Model file for the job. Use its own axes, mm. Face numbers are marked on the shaded views. Give positions to 0.01 mm unless a question says otherwise; leave off trailing zeros. Write each loop counter-clockwise with the first axis right and the second up, starting at its lowest first coordinate (ties: lowest second). Pieces come first, ordered by that corner, then holes.
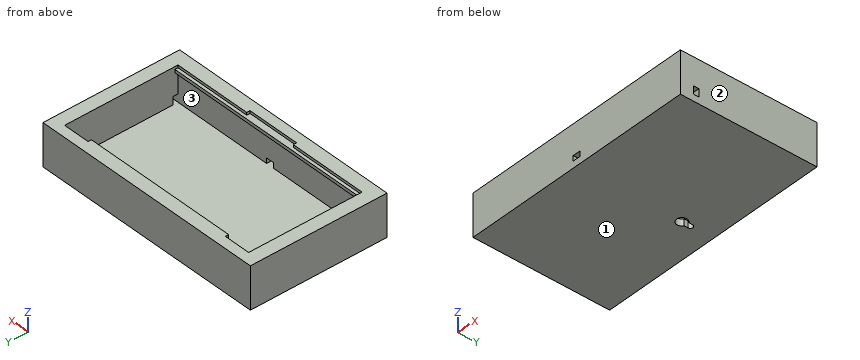
Autodesk Inventor part; units mm, degrees
ref_plane "YZ Plane" through (0, 0, 0) normal (1, 0, 0) x (0, 1, 0)
ref_plane "XZ Plane" through (0, 0, 0) normal (0, 1, 0) x (-1, 0, 0)
ref_plane "XY Plane" through (0, 0, 0) normal (0, 0, 1) x (1, 0, 0)
sketch "Sketch1" plane through (0, 0, 0) normal (0, 0, 1) x (1, 0, 0)
  line L0 (-100, -52.5) -> (100, -52.5)
  line L1 (100, -52.5) -> (100, 52.5)
  line L2 (100, 52.5) -> (-100, 52.5)
  line L3 (-100, 52.5) -> (-100, -52.5)
  line L4 (-100, -52.5) -> (100, 52.5) construction
  line L5 (100, -52.5) -> (-100, 52.5) construction
  line L6 (-112.7, 65.2) -> (112.7, 65.2)
  line L7 (112.7, 65.2) -> (112.7, -65.2)
  line L8 (112.7, -65.2) -> (-112.7, -65.2)
  line L9 (-112.7, -65.2) -> (-112.7, 65.2)
  point P0 (0, 0)
  dimension "d0" = 200
  dimension "d1" = 105
  dimension "d2" = 12.7
extrude "Extrusion1" add sketch "Sketch1" against normal blind 40
sketch "Sketch2" plane through (-100, 52.5, 0) normal (0, -1, 0) x (1, 0, 0)
  line L0 (200, -40) -> (0, -40)
  line L1 (0, 0) -> (0, -40)
  line L2 (200, -40) -> (0, -40)
  line L3 (0, -40) -> (0, -33.65)
  line L4 (0, -33.65) -> (200, -33.65)
  line L5 (200, -33.65) -> (200, -40)
  point P0 (100, 0)
  dimension "d5" = 6.35
extrude "Extrusion2" add sketch "Sketch2" along normal up to next
sketch "Sketch4" plane through (0, 0, -40) normal (0, 0, -1) x (-1, 0, 0)
  line L0 (112.7, 65.2) -> (-112.7, 65.2)
  line L1 (0, 65.2) -> (0, -65.2)
  line L2 (-112.7, -65.2) -> (112.7, -65.2)
  arc A0 (-2.5, 39.5301) -> (2.5, 39.5301) centre (0, 35.2) ccw
  line L3 (0, 35.2) -> (0, 43.2) construction
  line L4 (2.5, 39.5301) -> (2.5, 43.2)
  line L5 (-2.5, 43.2) -> (-2.5, 39.5301)
  arc A1 (2.5, 43.2) -> (-2.5, 43.2) centre (0, 43.2) ccw
  point P0 (0, 0)
  point P1 (0, 39.2)
  dimension "d14" = 10
  dimension "d15" = 5
  dimension "d17" = 30
  dimension "d18" = 8
extrude "Extrusion4" cut sketch "Sketch4" against normal through all
sketch "Sketch5" plane through (100, -52.5, 0) normal (-1, 0, 0) x (0, 0, 1)
  line L0 (-33.65, 105) -> (-33.65, 0)
  line L1 (0, 0) -> (-40, 0)
  line L2 (-33.65, 0) -> (-26.15, 0)
  line L3 (-26.15, 0) -> (-26.15, 5)
  line L4 (-26.15, 5) -> (-33.65, 5)
  line L5 (-33.65, 5) -> (-33.65, 0)
  point P0 (0, 52.5)
  dimension "d21" = 7.5
  dimension "d22" = 5
extrude "Extrusion5" cut sketch "Sketch5" against normal through all
sketch "Sketch6" plane through (-100, -52.5, 0) normal (1, 0, 0) x (0, 0, -1)
  line L0 (0, 0) -> (33.65, 0)
  line L1 (0, 0) -> (0, 105)
  line L2 (0, 105) -> (33.65, 105)
  line L3 (2.5, 0) -> (5.5, 0)
  line L4 (5.5, 0) -> (5.5, 3)
  line L5 (5.5, 3) -> (2.5, 3)
  line L6 (2.5, 3) -> (2.5, 0)
  point P0 (0, 52.5)
  point P1 (40, 0)
  point P2 (40, 105)
  dimension "d26" = 2.5
  dimension "d27" = 3
  dimension "d28" = 3
extrude "Extrusion6" add sketch "Sketch6" along normal up to next
sketch "Sketch7" plane through (0, 0, 0) normal (0, 0, 1) x (1, 0, 0)
  line L0 (112.7, -65.2) -> (-112.7, -65.2)
  line L1 (0, -65.2) -> (0, -52.5)
  line L2 (-100, -52.5) -> (112.7, -52.5)
  line L3 (-25.4, -55.675) -> (25.4, -55.675)
  line L4 (25.4, -55.675) -> (25.4, -52.5)
  line L5 (25.4, -52.5) -> (-25.4, -52.5)
  line L6 (-25.4, -52.5) -> (-25.4, -55.675)
  line L7 (-25.4, -55.675) -> (25.4, -52.5) construction
  line L8 (25.4, -55.675) -> (-25.4, -52.5) construction
  arc A0 (25.4, -55.675) -> (28.575, -52.5) centre (25.4, -52.5) ccw construction
  arc A1 (-28.575, -52.5) -> (-25.4, -55.675) centre (-25.4, -52.5) ccw construction
  point P0 (0, 0)
  point P1 (0, -54.0875)
  point P2 (100, -52.5)
  dimension "d32" = 50.8
  dimension "d33" = 3.175
extrude "Extrusion7" cut sketch "Sketch7" against normal up to surface (2.5 mm away)
sketch "Sketch8" plane through (0, 0, 0) normal (0, 0, 1) x (1, 0, 0)
  line L0 (-100, -52.5) -> (-100, 52.5)
  line L1 (-100, 52.5) -> (-74.6, 52.5)
  line L2 (-74.6, 52.5) -> (-74.6, 55.675)
  line L3 (-74.6, 55.675) -> (-100, 55.675)
  line L4 (-100, 55.675) -> (-100, 52.5)
  point P0 (0, 0)
  dimension "d36" = 25.4
  dimension "d37" = 3.175
extrude "Extrusion8" cut sketch "Sketch8" against normal blind 22.86
mirror "Mirror1" about plane through (0, 0, 0) normal (1, 0, 0) of "Extrusion8"
sketch "Sketch9" plane through (-100, -52.5, -33.65) normal (0, 1, 0) x (1, 0, 0)
  line L0 (0, 0) -> (212.7, 0)
  line L1 (96.2535, -5.0038) -> (103.7465, -5.0038)
  line L2 (103.7465, -5.0038) -> (103.7465, 0)
  line L3 (103.7465, 0) -> (96.2535, 0)
  line L4 (96.2535, 0) -> (96.2535, -5.0038)
  line L5 (212.7, 6.35) -> (-12.7, 6.35)
  line L6 (100, 6.35) -> (100, -33.65)
  line L7 (125.4, -33.65) -> (74.6, -33.65)
  point P0 (100, 0)
  point P1 (200, 0)
  dimension "d40" = 7.493
  dimension "d41" = 5.0038
extrude "Extrusion9" cut sketch "Sketch9" against normal through all
properties part number "housing"
1. Pull direction X, two halves, no side cores. Call the marked faces 1, 2 and 3: +X half, -X half, draft (parallel to the pull), parting line (faces both ways), or undercut.
Calculated:
face 1: draft
face 2: +X half
face 3: undercut
2. Slice it at B-B, the plane z = -9. Write the cut outline in (x, y) (3 decimals).
Calculated:
outline: (-112.7, -65.2) - (112.7, -65.2) - (112.7, 65.2) - (-112.7, 65.2) - close; hole (-100, -52.5) - (100, -52.5) - (100, 55.675) - (74.6, 55.675) - (74.6, 52.5) - (-74.6, 52.5) - (-74.6, 55.675) - (-100, 55.675) - close
3. Slice it at C-C, the plane y = -9.5. Write the cut outline in (x, z).
Calculated:
outline: (-112.7, -40) - (112.7, -40) - (112.7, 0) - (100, 0) - (100, -33.65) - (-100, -33.65) - (-100, 0) - (-112.7, 0) - close
4. Probe probe 1 along Y at (x, z) = (0, -35.25); probe 2 along X at (y, z) = (6, -19.5); probe 3 along Y at (x, z) = (94, -27.5). List the from-to ranges inside material, lowest first.
Calculated:
probe 1: y = -65.2 to 30.2, 45.7 to 65.2
probe 2: x = -112.7 to -100, 100 to 112.7
probe 3: y = -65.2 to -52.5, 52.5 to 65.2
5. Pin check, flat tips, straight feed: P1, Ø1.9, axis at x = -12, y = -54, coming from the +Z side; P2, Ø1, axis at x = -38.5, y = -46.5, coming from the +Z side; P3, Ø1.6, axis at x = 89.5, y = 54, coming from the +Z side. Stop position of each tip, or through.
Calculated:
P1: stops at z = -2.5
P2: stops at z = -33.65
P3: stops at z = -22.86
6. Slice it at A-A, the plane y = 35.2. Write the cut outline in (x, z), and give its area (3 significant figures).
Calculated:
outline: (-112.7, -40) - (-5, -40) - (-5, -33.65) - (-100, -33.65) - (-100, 0) - (-112.7, 0) - close; (5, -40) - (112.7, -40) - (112.7, 0) - (100, 0) - (100, -33.65) - (5, -33.65) - close
area: 2,220 mm2
